```python
from build123d import *

# Parameters (mm, degrees)
EXTRUDE_1_DEPTH          = 3.1
EXTRUDE_2_DEPTH          = 0.8
FILLET_1_SIZE            = 0.3
FILLET_1_SIZE_2          = 1.8
SKETCH_3_R               = 1
SKETCH_3_R_2             = 1.096749421
EXTRUDE_3_DEPTH          = 1.05
FILLET_5_R               = 0.9
CUT_EXTRUDE_2_DEPTH      = 82.307539193
CUT_EXTRUDE_2_DEPTH_BACK = 82.307539193
SKETCH_7_W               = 5.8
SKETCH_7_H               = 24.900002621
FILLET_6_R               = 1


with BuildPart() as part:
    # 草图1 → 凸台-拉伸1 (new body)
    with BuildSketch(Plane.XY):
        with BuildLine():
            Line((-1.3, -78.273), (-1.3, -61.672998253))
            ThreePointArc((-1.3, -61.672998253), (0.6, -59.772998253), (2.5, -61.672998253))
            Line((2.5, -61.672998253), (2.5, -78.273))
            ThreePointArc((2.5, -78.273), (0.6, -80.173), (-1.3, -78.273))
        make_face()
    extrude(amount=EXTRUDE_1_DEPTH)

    # 草图2 → 凸台-拉伸2 (add)
    with BuildSketch(Plane(origin=(0, 0, 0), x_dir=(-1, 0, 0), z_dir=(0, 0, -1))):
        with BuildLine():
            Line((2.3, -78.273), (2.3, -61.672998253))
            ThreePointArc((2.3, -61.672998253), (-0.6, -58.772998253), (-3.5, -61.672998253))
            Line((-3.5, -61.672998253), (-3.5, -78.273))
            ThreePointArc((-3.5, -78.273), (-0.6, -81.173), (2.3, -78.273))
        make_face()
    extrude(amount=-EXTRUDE_2_DEPTH)

    # 圆角1
    # an asymmetric fillet: 1.8, 0.3 mm, written as the material it takes off along each edge
    with BuildSketch(Plane(origin=(2.5, -61.672998253, 3.1), x_dir=(0, 0, -1), z_dir=(0, -1, 0)), Plane(origin=(-1.3, -78.273, 3.1), x_dir=(0, 0, -1), z_dir=(0, 1, 0))) as fillet_1_piece_1:
        with BuildLine():
            Bezier((FILLET_1_SIZE, 0), (0, 0), (0, -FILLET_1_SIZE_2), weights=[1, 0.707106781, 1])
            Line((0, -FILLET_1_SIZE_2), (0, 0))
            Line((0, 0), (FILLET_1_SIZE, 0))
        make_face()
    extrude(amount=16.600001747, mode=Mode.SUBTRACT)
    with BuildSketch(Plane(origin=(0.6, -61.672998253, 3.1), x_dir=(-1, 0, 0), z_dir=(0, -1, 0))) as fillet_1_piece_2:
        with BuildLine():
            Bezier((1.9, FILLET_1_SIZE), (1.9, 0), (1.9 - FILLET_1_SIZE_2, 0), weights=[1, 0.707106781, 1])
            Line((1.9 - FILLET_1_SIZE_2, 0), (1.9, 0))
            Line((1.9, 0), (1.9, FILLET_1_SIZE))
        make_face()
    revolve(axis=Axis((0.6, -61.672998253, 3.1), (0, 0, -1)), revolution_arc=180, mode=Mode.SUBTRACT)
    with BuildSketch(Plane(origin=(0.6, -78.273, 3.1), x_dir=(1, 0, 0), z_dir=(0, 1, 0))) as fillet_1_piece_3:
        with BuildLine():
            Bezier((1.9, FILLET_1_SIZE), (1.9, 0), (1.9 - FILLET_1_SIZE_2, 0), weights=[1, 0.707106781, 1])
            Line((1.9 - FILLET_1_SIZE_2, 0), (1.9, 0))
            Line((1.9, 0), (1.9, FILLET_1_SIZE))
        make_face()
    revolve(axis=Axis((0.6, -78.273, 3.1), (0, 0, -1)), revolution_arc=180, mode=Mode.SUBTRACT)

    # 草图3 → 凸台-拉伸3 (add)
    with BuildSketch(Plane(origin=(0, 0, 0), x_dir=(-1, 0, 0), z_dir=(0, 0, -1))):
        with Locations(Location((-0.6, -61.672998253, 0), (0, 0, 180))):
            Circle(SKETCH_3_R)
        with Locations(Location((-0.6, -69.972999126, 0), (0, 0, 180))):
            Circle(SKETCH_3_R_2)
        with Locations(Location((-0.6, -78.273, 0), (0, 0, 180))):
            Circle(SKETCH_3_R_2)
    extrude(amount=EXTRUDE_3_DEPTH)

    # 圆角5
    fillet_5_edges = [part.edges().sort_by_distance(p)[0] for p in [
        (-0.4, -61.672998253, 0),
        (-0.496749421, -69.972999126, 0),
        (-0.496749421, -78.273, 0),
    ]]
    fillet(fillet_5_edges, radius=FILLET_5_R)

    # 草图7 → 切除-拉伸2 (cut, two sides: drawn at the far end of the back side and taken through both)
    with BuildSketch(Plane(origin=(0, 0, 0), x_dir=(-1, 0, 0), z_dir=(0, 0, -1)).offset(-CUT_EXTRUDE_2_DEPTH_BACK)):
        with Locations((-0.6, -61.672998253)):
            Rectangle(SKETCH_7_W, SKETCH_7_H)
    extrude(amount=CUT_EXTRUDE_2_DEPTH + CUT_EXTRUDE_2_DEPTH_BACK, mode=Mode.SUBTRACT)

    # 圆角6
    fillet_6_edges = [part.edges().sort_by_distance(p)[0] for p in [
        (-2.3, -74.122999563, 0.4),
        (3.5, -74.122999563, 0.4),
    ]]
    fillet(fillet_6_edges, radius=FILLET_6_R)


solid = part.part
```
Geometry check sheet. Reference: the model listing, model coordinates, mm. A direction names the side the tool comes from. Give positions to 0.01 mm unless a question says otherwise; leave off trailing zeros. Order: outer loops, then holes, each group sorted by start corner. A loop starts at its lowest first (then second) coordinate and runs counter-clockwise, first axis right, second up.
1. Section check B-B, the plane y = -80.5. Enter the section's corners in (x, z).
2. Access from +Z, -Z, +X, -X, +Y, -Y to the whole of each face (thin tool, end or side, straight path). Record for faces 1 (the face through (-1.3, -76, 2)), 2 (the face through (2.5, -76, 2)), 3 (the face through (1, -76, 0)), 4 (the face through (0.642, -80.173, 1.786)), 5 (the face through (1, -74.123, 2)).
3. Gauge pin test, flat ends, axial feed: pin 1 Ø2 at (y, z) = (-75.5, 2) entering from -X; pin 2 Ø1 at (y, z) = (-77, 2.5) entering from +X; pin 3 Ø2 at (y, z) = (-79.5, 0.5) entering from -X. Record the tip position at first contact, or that the pin passes through.
4. Section check A-A, the plane z = 1.8. Enter the section's corners in (x, y).
5. Thickness scan on L1, parallel to X at y = -76.25, z = 1.6; L2, parallel to Z at x = 3.15, y = -75.5; L3, parallel to Y at x = 0.5, z = 1.05. Record the ranges inside material, lowest first.
Values follow:
1. outline: (-1.26, 0) - (2.46, 0) - (2.46, 0.8) - (-1.26, 0.8) - close
2. face 1: +Z, -X, +Y, -Y
2. face 2: +Z, +X, +Y, -Y
2. face 3: -Z
2. face 4: +Z, -Y
2. face 5: +Z, -Z, +X, -X, +Y
3. pin 1: stops at x = -1.3
3. pin 2: stops at x = 2.5
3. pin 3: stops at x = -2.29
4. outline: (-1.3, -78.27) arc R1.9 ccw to (2.5, -78.27) - (2.5, -74.12) - (-1.3, -74.12) - close
5. L1: x = -1.3 to 2.5
5. L2: z = 0 to 0.8
5. L3: y = -80.17 to -74.12
